Verification items for the finished model (mm, model axes). A direction names the side the tool comes from. Coordinates: 2 decimals unless noted, no trailing zeros. Write each loop counter-clockwise with the first axis right and the second up, starting at its lowest first coordinate (ties: lowest second). Pieces come first, ordered by that corner, then holes. Notation, with made-up numbers: (8, 32.5) -> (63, 32.5) arc R20 cw to (63, 51.5) -> close; hole circle Ø4 at (68, -26). An arc over 180 degrees is marked (long way). Use CSV: the item, a comma, the result in double quotes.
```python
from build123d import *


with BuildPart() as part:
    # Sketch1 → Revolve1 (revolve)
    with BuildSketch(Plane.XY, mode=Mode.PRIVATE) as revolve1_sk:
        Polygon((0, 0), (1.9812, 0), (1.9812, 9.8806), (2.38125, 9.8806), (2.38125, 19.4818), (4.7371, 19.4818), (4.7371, 25.0444), (2.7686, 25.0444), (2.7686, 32.4866), (1.9177, 32.4866), (1.9177, 38.8366), (2.794, 38.8366), (2.794, 40.4241), (0.3175, 44.9834), (0, 44.9834), align=None)
    revolve(revolve1_sk.sketch.rotate(Axis((0, 0, 0), (0, 1, 0)), 90), axis=Axis((0, 0, 0), (0, 1, 0)))  # turned: the seam where the file's is


solid = part.part
```
1) Mould release check, pull along Y, two halves, no side actions. Record for faces 4 (the flat face through (0, 0, 0)), 5 (the cylindrical face through (1.7, 39.641, 2.217)), 6 (the cylindrical face through (-1.9, 35.71, 0.25)): released by +Y, released by -Y, zero draft, split by the parting line, or undercut.
Return value:
face 4,"released by -Y"
face 5,"zero draft"
face 6,"undercut"
2) Scan lines: L1, parallel to Z at x = 2, y = 27; L2, parallel to Y at x = -2.5, z = 3.25; L3, parallel to X at y = 37, z = 1.5. Record each from-to range of solid material in increasing order.
Return value:
L1,"-1.91 to 1.91"
L2,"19.48 to 25.04"
L3,"-1.19 to 1.19"
3) Cross-section at A-A (y = 13). Record the boundary of the cut face in (x, z), plus the area to 3 significant figures.
Return value:
outline,"circle Ø4.76 at (0, 0)"
area,"17.8 mm2"
4) Set-up check for faces 1 (the cylindrical face through (4.624, 22.302, 1.027)), 2 (the flat face through (2, 19.482, 2)), 3 (the flat face through (-1, 32.487, -2)): record each of +Z, -Z, +X, -X, +Y, -Y from which the full face is reachable in a straight line by a thin tool's end or side.
Return value:
face 1,"+Y, -Y"
face 2,"-Y"
face 3,"none"
5) Gauge pin test, flat ends, axial feed: pin 1 (3 mm diameter, centred on x = 1, y = 35, fed in from +Z); pin 2 (2 mm diameter, centred on y = 34.5, z = -3.5, fed in from -X); pin 3 (1.5 mm diameter, centred on y = 17, z = 0.5, fed in from +X); pin 4 (3 mm diameter, centred on x = -2, z = -0.5, fed in from +Y). Record the tip position at first contact, or that the pin passes through.
Return value:
pin 1,"z = 1.92"
pin 2,"through"
pin 3,"x = 2.38"
pin 4,"y = 44.53"
6) Cross-section at C-C (y = 22). Record the boundary of the cut face in (x, z).
Return value:
outline,"circle Ø9.47 at (0, 0)"
7) Cross-section at B-B (x = -3.25). Record the boundary of the cut face in (y, z).
Return value:
outline,"(19.48, -3.45) -> (25.04, -3.45) -> (25.04, 3.45) -> (19.48, 3.45) -> close"
